```python
from build123d import *

# Parameters (mm, degrees)
ESQUISSE1_R             = 6
BOSS_EXTRU_1_DEPTH      = 25
ENL_V_MAT_EXTRU_1_REACH = 54.097
ESQUISSE2_R             = 3.3
ESQUISSE3_R             = 5.4
ENL_V_MAT_EXTRU_2_DEPTH = 5
ESQUISSE4_W             = 34
ESQUISSE4_H             = 34.910709465
ESQUISSE4_R             = 6
BOSS_EXTRU_2_DEPTH      = 5


with BuildPart() as part:
    # Esquisse1 → Boss.-Extru.1 (new body)
    with BuildSketch(Plane.XY):
        Polygon((-27.861974124, -13.935926773), (32.138025876, -13.935926773), (32.138025876, 18.564073227), (19.138025876, 18.564073227), (19.138025876, 29.064073227), (-14.861974124, 29.064073227), (-14.861974124, 18.564073227), (-27.861974124, 18.564073227), align=None)
        with Locations((2.138025876, 11.064073227)):
            Circle(ESQUISSE1_R, mode=Mode.SUBTRACT)
    extrude(amount=BOSS_EXTRU_1_DEPTH)

    # Esquisse2 → Enlèv. mat.-Extru.1 (cut, up to next)
    with BuildSketch(Plane(origin=(0, 18.564073227, 0), x_dir=(1, 0, 0), z_dir=(0, 1, 0)), mode=Mode.PRIVATE) as enl_v_mat_extru_1_sk1:
        with Locations(Location((25.138025876, -19, 0), (0, 0, 270))):
            Circle(ESQUISSE2_R)
    enl_v_mat_extru_1_tool1 = extrude(enl_v_mat_extru_1_sk1.sketch, amount=-ENL_V_MAT_EXTRU_1_REACH, mode=Mode.PRIVATE) & part.part
    # Esquisse2 → Enlèv. mat.-Extru.1 (cut, up to next)
    with BuildSketch(Plane(origin=(0, 18.564073227, 0), x_dir=(1, 0, 0), z_dir=(0, 1, 0)), mode=Mode.PRIVATE) as enl_v_mat_extru_1_sk2:
        with Locations(Location((25.138025876, -6, 0), (0, 0, 270))):
            Circle(ESQUISSE2_R)
    enl_v_mat_extru_1_tool2 = extrude(enl_v_mat_extru_1_sk2.sketch, amount=-ENL_V_MAT_EXTRU_1_REACH, mode=Mode.PRIVATE) & part.part
    # Esquisse2 → Enlèv. mat.-Extru.1 (cut, up to next)
    with BuildSketch(Plane(origin=(0, 18.564073227, 0), x_dir=(1, 0, 0), z_dir=(0, 1, 0)), mode=Mode.PRIVATE) as enl_v_mat_extru_1_sk3:
        with Locations(Location((-20.861974124, -19, 0), (0, 0, 270))):
            Circle(ESQUISSE2_R)
    enl_v_mat_extru_1_tool3 = extrude(enl_v_mat_extru_1_sk3.sketch, amount=-ENL_V_MAT_EXTRU_1_REACH, mode=Mode.PRIVATE) & part.part
    # Esquisse2 → Enlèv. mat.-Extru.1 (cut, up to next)
    with BuildSketch(Plane(origin=(0, 18.564073227, 0), x_dir=(1, 0, 0), z_dir=(0, 1, 0)), mode=Mode.PRIVATE) as enl_v_mat_extru_1_sk4:
        with Locations(Location((-20.861974124, -6, 0), (0, 0, 270))):
            Circle(ESQUISSE2_R)
    enl_v_mat_extru_1_tool4 = extrude(enl_v_mat_extru_1_sk4.sketch, amount=-ENL_V_MAT_EXTRU_1_REACH, mode=Mode.PRIVATE) & part.part
    add(enl_v_mat_extru_1_tool1.solids().sort_by_distance((25.138026, 18.564073, 19))[0], mode=Mode.SUBTRACT)
    add(enl_v_mat_extru_1_tool2.solids().sort_by_distance((25.138026, 18.564073, 6))[0], mode=Mode.SUBTRACT)
    add(enl_v_mat_extru_1_tool3.solids().sort_by_distance((-20.861974, 18.564073, 19))[0], mode=Mode.SUBTRACT)
    add(enl_v_mat_extru_1_tool4.solids().sort_by_distance((-20.861974, 18.564073, 6))[0], mode=Mode.SUBTRACT)

    # Esquisse3 → Enlèv. mat.-Extru.2 (cut)
    with BuildSketch(Plane(origin=(0, 18.564073227, 0), x_dir=(1, 0, 0), z_dir=(0, 1, 0))):
        with Locations(Location((25.138025876, -19, 0), (0, 0, 270))):
            Circle(ESQUISSE3_R)
        with Locations(Location((25.138025876, -6, 0), (0, 0, 270))):
            Circle(ESQUISSE3_R)
        with Locations(Location((-20.861974124, -6, 0), (0, 0, 270))):
            Circle(ESQUISSE3_R)
        with Locations(Location((-20.861974124, -19, 0), (0, 0, 270))):
            Circle(ESQUISSE3_R)
    extrude(amount=-ENL_V_MAT_EXTRU_2_DEPTH, mode=Mode.SUBTRACT)

    # Esquisse4 → Boss.-Extru.2 (add)
    with BuildSketch(Plane.XY.offset(25)):
        with Locations((2.138025876, 11.064073226)):
            Rectangle(ESQUISSE4_W, ESQUISSE4_H)
        with Locations((2.138025876, 11.064073227)):
            Circle(ESQUISSE4_R, mode=Mode.SUBTRACT)
    extrude(amount=BOSS_EXTRU_2_DEPTH)


solid = part.part
```
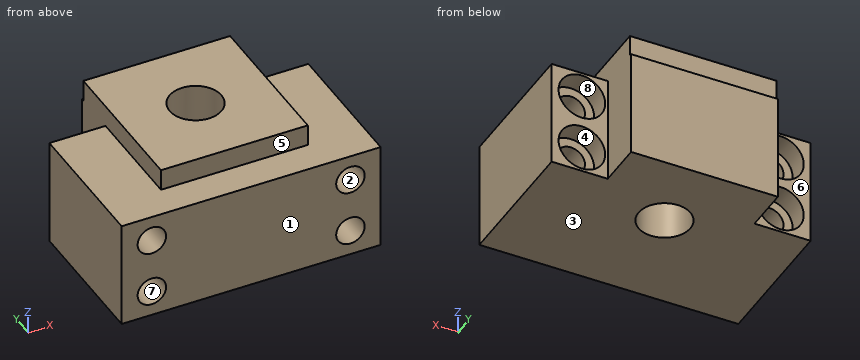
Read the model definition and answer for the solid it produces. Units are mm, in the model's axes. Face numbers are marked on the shaded views. A direction names the side the tool comes from. Round coordinates to 2 decimals unless told otherwise and drop trailing zeros. Write each loop counter-clockwise with the first axis right and the second up, starting at its lowest first coordinate (ties: lowest second). Pieces come first, ordered by that corner, then holes. Notation, with made-up numbers: (18, 74) - (53, 74) arc R24 ccw to (53, 106) - close; hole circle Ø1 at (-36.75, -12.75). An arc over 180 degrees is marked (long way). One line per item, written item: value.
Q1. Which of the six approach directions +Z, -Z, +X, -X, +Y, -Y give full straight-line access (tool end or side, diameter ignored) to the marked faces 5, 6, 7 and 8?
The answers:
face 5: +Z, +X, -X, -Y
face 6: +Z, -Z, -X, +Y
face 7: +Y, -Y
face 8: +Y
Q2. Find section B-B (z = 6). Determine the outline of the cut face in (x, y), and give its area (3 significant figures).
The answers:
outline: (-27.86, -13.94) - (-24.16, -13.94) - (-24.16, 13.56) - (-26.26, 13.56) - (-26.26, 18.56) - (-27.86, 18.56) - close; (-17.56, -13.94) - (21.84, -13.94) - (21.84, 13.56) - (19.74, 13.56) - (19.74, 18.56) - (19.14, 18.56) - (19.14, 29.06) - (-14.86, 29.06) - (-14.86, 18.56) - (-15.46, 18.56) - (-15.46, 13.56) - (-17.56, 13.56) - close; (28.44, -13.94) - (32.14, -13.94) - (32.14, 18.56) - (30.54, 18.56) - (30.54, 13.56) - (28.44, 13.56) - close; hole circle Ø12 at (2.14, 11.06)
area: 1,720 mm2
Q3. Find section D-D (z = 2). Determine the outline of the cut face in (x, y), and give its area (3 significant figures).
The answers:
outline: (-27.86, -13.94) - (32.14, -13.94) - (32.14, 18.56) - (28.77, 18.56) - (28.77, 13.56) - (21.51, 13.56) - (21.51, 18.56) - (19.14, 18.56) - (19.14, 29.06) - (-14.86, 29.06) - (-14.86, 18.56) - (-17.23, 18.56) - (-17.23, 13.56) - (-24.49, 13.56) - (-24.49, 18.56) - (-27.86, 18.56) - close; hole circle Ø12 at (2.14, 11.06)
area: 2,120 mm2
Q4. For a pull along Z with two mould halves and no side action, classify the marked faces 1, 2, 3 and 4 as pulls with the +Z half, pulls with the -Z half, needs draft (parallel to the pull), parting line crosses it, or undercut.
The answers:
face 1: needs draft
face 2: undercut
face 3: pulls with the -Z half
face 4: undercut
Q5. Straight lines are drawn through the part: line 1 (X direction, y = 4, z = 19); line 2 (X direction, y = 14.5, z = 14.5); line 3 (X direction, y = 15.7, z = 19). For each, find the intervals that lie inside material, in ascending order. Write a range as from..to.
The answers:
line 1: x = -27.86..-24.16, -17.56..21.84, 28.44..32.14
line 2: x = -27.86..-23.85, -17.88..-2.78, 7.06..22.15, 28.12..32.14
line 3: x = -27.86..-26.26, -15.46..-1.67, 5.95..19.74, 30.54..32.14
Q6. Each of these flat-tipped pins is pushed along its axis until it touches: P1, Ø10.5, axis at x = -20.86, z = 6, coming from the +Y side; P2, Ø5.5, axis at x = -18.5, z = 20.5, coming from the +Y side; P3, Ø19, axis at x = 2.14, y = 11.06, coming from the -Z side; P4, Ø5, axis at x = 4, y = 8.5, coming from the +Z side. Where does it stop, or does it pass through?
The answers:
P1: stops at y = 13.56
P2: stops at y = 18.56
P3: stops at z = 0
P4: passes through
Q7. Find section A-A (y = 8.5). Determine the outline of the cut face in (x, z), and give its area (3 significant figures).
The answers:
outline: (-27.86, 0) - (-3.29, 0) - (-3.29, 30) - (-14.86, 30) - (-14.86, 25) - (-27.86, 25) - close; (7.56, 0) - (32.14, 0) - (32.14, 25) - (19.14, 25) - (19.14, 30) - (7.56, 30) - close; hole circle Ø6.6 at (-20.86, 6); hole circle Ø6.6 at (-20.86, 19); hole circle Ø6.6 at (25.14, 6); hole circle Ø6.6 at (25.14, 19)
area: 1,210 mm2
Q8. Find section C-C (x = -23.5). Determine the outline of the cut face in (y, z).
The answers:
outline: (-13.94, 0) - (18.56, 0) - (18.56, 1.29) - (13.56, 1.29) - (13.56, 4.02) - (-13.94, 4.02) - close; (-13.94, 7.98) - (13.56, 7.98) - (13.56, 10.71) - (18.56, 10.71) - (18.56, 14.29) - (13.56, 14.29) - (13.56, 17.02) - (-13.94, 17.02) - close; (-13.94, 20.98) - (13.56, 20.98) - (13.56, 23.71) - (18.56, 23.71) - (18.56, 25) - (-13.94, 25) - close
